Check sheet for the modelled part. Datum: model origin and axes. Units: mm. A direction names the side the tool comes from. Coordinates: 2 decimals unless noted, no trailing zeros. Write each loop counter-clockwise with the first axis right and the second up, starting at its lowest first coordinate (ties: lowest second). Pieces come first, ordered by that corner, then holes. Notation, with made-up numbers: (10.5, 44) -> (40.5, 44) arc R24 cw to (40.5, 82) -> close; hole circle Ø1 at (77, -20.75). An arc over 180 degrees is marked (long way). One line per item, written item: value. Start each with the question number.
1) Sectioned sample at B-B on y = 0.5. Enter the section's corners in (x, z).
2) Scan lines: line 1 along Y through (x, z) = (-7, 2.3); line 2 along Y through (x, z) = (14.75, 1.4); line 3 along X through (y, z) = (11, 1.25). Record each from-to range of solid material in increasing order. Write a range as [from, to].
3) Gauge pin test, flat end, axial feed: P1, Ø3, axis at x = -7, y = 0.5, coming from the +Z side (1 decimal). Record the tip position at first contact, or that the pin passes through.
4) Sectioned sample at D-D on z = 1. Give the number of separate pieces and of enclosed holes in the cut face, plus the area to 3 significant figures.
5) Set-up check for faces 1 (the flat face through (22.5, 3, 1)), 2 (the flat face through (2.254, 11.792, 1.479)): record each of +Z, -Z, +X, -X, +Y, -Y from which the full face is reachable in a straight line by a thin tool's end or side.
6) Sectioned sample at A-A on x = -7. Enter the section's corners in (y, z).
7) Draft check along Y on faces 3 (the flat face through (-2.27, 7.19, 1.48)), 4 (the flat face through (2.245, 7.137, 1.479)), 5 (the cylindrical face through (21.359, -12.497, 1.521)), 6 (the cylindrical face through (-21.297, 18.159, 1.521)). Enter one of: +Y half, -Y half, draft (parallel to the pull), parting line (faces both ways), or undercut.
8) Sectioned sample at C-C on x = 14.75. Enter the section's corners in (y, z).
```python
from build123d import *

# Parameters (mm, degrees)
SKETCH1_R                                    = 1.8
BOSS_EXTRUDE1_DEPTH                          = 3
FILLET1_R                                    = 4
CSK_FOR_M3_COUNTERSUNK_FLAT_HEAD_SCR_2_COUNT = 2
CSK_FOR_M3_COUNTERSUNK_FLAT_HEAD_SCR_2_PITCH = 7


with BuildPart() as part:
    # Sketch1 → Boss-Extrude1 (new body)
    with BuildSketch(Plane.XY):
        Polygon((22.5, 19.3), (-22.5, 19.3), (-22.5, -9.7), (-22.5, -13.7), (22.5, -13.7), (22.5, -9.7), align=None)
        with Locations((14.75, 16)):
            Circle(SKETCH1_R, mode=Mode.SUBTRACT)
        with Locations((-14.75, 16)):
            Circle(SKETCH1_R, mode=Mode.SUBTRACT)
        with BuildLine():
            Line((-3.479994944, 4.879643035), (-1.504454613, 4.879643035))
            Line((-1.504454613, 4.879643035), (-0.716662457, 6.696078227))
            add(Edge.make_bspline(
                [(-0.716662457, 6.696078227), (-0.662988728, 6.823847603), (-0.558253832, 7.073167199), (-0.407159323, 7.448475347), (-0.260246479, 7.833509844), (-0.163053085, 8.096372908), (-0.1123781, 8.233425246)],
                knots=[0, 0, 0, 0, 0.000415753, 0.000811269, 0.001213674, 0.001652036, 0.001652036, 0.001652036, 0.001652036], degree=3))
            Line((-0.1123781, 8.233425246), (-0.086428732, 8.234214033))
            add(Edge.make_bspline(
                [(-0.086428732, 8.234214033), (0.016216114, 7.980645356), (0.223344012, 7.468966992), (0.443707362, 6.962847127), (0.554866869, 6.707541356)],
                knots=[0, 0, 0, 0, 0.000820631, 0.001655958, 0.001655958, 0.001655958, 0.001655958], degree=3))
            Line((0.554866869, 6.707541356), (1.392196546, 4.879643035))
            Line((1.392196546, 4.879643035), (3.391976635, 4.879643035))
            Line((3.391976635, 4.879643035), (1.064959804, 9.457455895))
            Line((1.064959804, 9.457455895), (3.476699187, 14.192976369))
            Line((3.476699187, 14.192976369), (1.513395339, 14.192976369))
            Line((1.513395339, 14.192976369), (0.749842942, 12.400503146))
            add(Edge.make_bspline(
                [(0.749842942, 12.400503146), (0.683388417, 12.247174796), (0.555592527, 11.952315518), (0.374121285, 11.520725487), (0.206338492, 11.105720206), (0.107367824, 10.829588001), (0.057944958, 10.691696187)],
                knots=[0, 0, 0, 0, 0.000501324, 0.000964075, 0.001404587, 0.001843989, 0.001843989, 0.001843989, 0.001843989], degree=3))
            Line((0.057944958, 10.691696187), (0.022650182, 10.692809062))
            add(Edge.make_bspline(
                [(0.022650182, 10.692809062), (-0.035080758, 10.828878889), (-0.150655612, 11.101284822), (-0.329423009, 11.514746078), (-0.526398165, 11.943735097), (-0.667307197, 12.235388249), (-0.740993098, 12.387903135)],
                knots=[0, 0, 0, 0, 0.000443432, 0.000887733, 0.001351306, 0.001859446, 0.001859446, 0.001859446, 0.001859446], degree=3))
            Line((-0.740993098, 12.387903135), (-1.577173889, 14.192976369))
            Line((-1.577173889, 14.192976369), (-3.589073858, 14.192976369))
            Line((-3.589073858, 14.192976369), (-1.092378716, 9.445344589))
            Line((-1.092378716, 9.445344589), (-3.479994944, 4.879643035))
        make_face(mode=Mode.SUBTRACT)
    extrude(amount=BOSS_EXTRUDE1_DEPTH)

    # Fillet1
    fillet1_edges = [part.edges().sort_by_distance(p)[0] for p in [
        (-22.5, 19.3, 1.5),
        (22.5, 19.3, 1.5),
        (22.5, -13.7, 1.5),
        (-22.5, -13.7, 1.5),
    ]]
    fillet(fillet1_edges, radius=FILLET1_R)

    # Sketch6 → CSK for M3 Countersunk Flat Head Screw1 (revolve, cut)
    with BuildSketch(Plane(origin=(-7, -6.5, 0), x_dir=(0, 1, 0), z_dir=(1, 0, 0))):
        Polygon((0, 0), (0, 3), (1.7, 3), (1.7, 1.45), (3.15, 0), align=None)
    csk_for_m3_countersunk_flat_head_screw1 = revolve(axis=Axis((-7, -6.5, -6.35), (0, 0, 1)), mode=Mode.SUBTRACT)

    # CSK for M3 Countersunk Flat Head Scr 2: CSK for M3 Countersunk Flat Head Screw1 ×2
    with Locations(*[(0, i * CSK_FOR_M3_COUNTERSUNK_FLAT_HEAD_SCR_2_PITCH, 0) for i in range(1, CSK_FOR_M3_COUNTERSUNK_FLAT_HEAD_SCR_2_COUNT)]):
        add(csk_for_m3_countersunk_flat_head_screw1, mode=Mode.SUBTRACT)


solid = part.part
```
Answers:
1. outline: (-22.5, 0) -> (-10.15, 0) -> (-8.7, 1.45) -> (-8.7, 3) -> (-22.5, 3) -> close; (-5.3, 1.45) -> (-3.85, 0) -> (22.5, 0) -> (22.5, 3) -> (-5.3, 3) -> close
2. line 1: y = [-13.7, -8.2], [-4.8, -1.2], [2.2, 19.3]
2. line 2: y = [-13.7, 14.2], [17.8, 19.3]
2. line 3: x = [-22.5, -1.91], [-0.11, 0.17], [1.85, 22.5]
3. P1: passes through
4. separate pieces: 1
4. enclosed holes: 5
4. area: 1,390 mm2
5. face 1: +Z, -Z, +X, +Y, -Y
5. face 2: +Z, -Z
6. outline: (-13.7, 0) -> (-9.65, 0) -> (-8.2, 1.45) -> (-8.2, 3) -> (-13.7, 3) -> close; (-4.8, 1.45) -> (-3.35, 0) -> (-2.65, 0) -> (-1.2, 1.45) -> (-1.2, 3) -> (-4.8, 3) -> close; (2.2, 1.45) -> (3.65, 0) -> (19.3, 0) -> (19.3, 3) -> (2.2, 3) -> close
7. face 3: undercut
7. face 4: undercut
7. face 5: -Y half
7. face 6: +Y half
8. outline: (-13.7, 0) -> (14.2, 0) -> (14.2, 3) -> (-13.7, 3) -> close; (17.8, 0) -> (19.3, 0) -> (19.3, 3) -> (17.8, 3) -> close
